Input: part model. Units: mm. Frame: model coordinates. A direction names the side the tool comes from. Coordinates: 2 decimals unless noted, no trailing zeros. Loops run counter-clockwise (first coordinate to the right, second up) from the corner with the lowest first, then second, coordinate; pieces in that order, holes last.
Autodesk Inventor part; units mm, degrees
ref_plane "YZ Plane" through (0, 0, 0) normal (1, 0, 0) x (0, 1, 0)
ref_plane "XZ Plane" through (0, 0, 0) normal (0, 1, 0) x (-1, 0, 0)
ref_plane "XY Plane" through (0, 0, 0) normal (0, 0, 1) x (1, 0, 0)
sketch "Sketch1" plane through (0, 0, 0) normal (0, 1, 0) x (-1, 0, 0)
  line L0 (0, 0) -> (14, 0)
  line L1 (14, 0) -> (14, -8.4)
  line L2 (14, -8.4) -> (0, -8.4)
  line L3 (0, -8.4) -> (0, 0)
  dimension "d0" = 8.4
  dimension "d1" = 14
extrude "Extrusion1" add sketch "Sketch1" along normal blind 2.5
sketch "Sketch2" plane through (0, 2.5, 0) normal (0, 1, 0) x (1, 0, 0)
  line L0 (-14, 2.85) -> (-5, 2.85)
  line L1 (-5, 5.55) -> (-14, 5.55)
  line L2 (-14, 5.55) -> (-14, 2.85)
  line L3 (-14, 8.4) -> (-14, 0)
  line L4 (-5, 2.85) -> (-5, 0)
  line L5 (-14, 0) -> (0, 0)
  line L6 (-5, 0) -> (0, 0)
  line L7 (0, 0) -> (0, 8.4)
  line L8 (0, 0) -> (0, 8.4)
  line L9 (-5, 5.55) -> (-5, 8.4)
  line L10 (0, 8.4) -> (-14, 8.4)
  point P0 (-14, 4.2)
  point P1 (-14, 4.2)
  point P2 (-5, 1.425)
  point P3 (-5, 6.975)
  dimension "d4" = 9
extrude "Extrusion2" add sketch "Sketch2" along normal blind 10 contours L2 L1 L9 L10 L7 L5 L4 L0
sketch "Sketch3" plane through (0, 0, 0) normal (0, -1, 0) x (1, 0, 0)
  line L0 (0, -29.6) -> (8, -29.6)
  line L1 (8, -29.6) -> (8, 21.2)
  line L2 (8, 21.2) -> (0, 21.2)
  line L3 (0, 21.2) -> (0, -29.6)
  line L4 (0, 0) -> (0, -8.4)
  point P0 (8, -4.2)
  point P1 (0, -4.2)
  point P2 (0, -4.2)
  dimension "d8" = 50.8
  dimension "d9" = 8
extrude "Extrusion3" add sketch "Sketch3" against normal up to surface (12.5 mm away)
sketch "Sketch4" plane through (0, 12.5, 0) normal (0, 1, 0) x (1, 0, 0)
  line L0 (16.1115, -33.9) -> (-34.6885, -33.9)
  line L1 (-34.6885, -33.9) -> (-34.6885, 42.3)
  line L2 (-34.6885, 42.3) -> (16.1115, 42.3)
  line L3 (16.1115, 42.3) -> (16.1115, -33.9)
  line L4 (8, 29.6) -> (8, -21.2)
  point P0 (0, 0)
  point P1 (16.1115, 4.2)
  point P2 (8, 4.2)
  dimension "d12" = 50.8
  dimension "d13" = 76.2
extrude "Extrusion4" add sketch "Sketch4" along normal blind 5
Item 1: Line query: L1, parallel to X at y = 10.5, z = 2.5; L2, parallel to Y at x = 13, z = 22; L3, parallel to X at y = 9.25, z = -7. Output: solid intervals per line, ascending.
Result:
L1: x = 0 to 8
L2: y = 12.5 to 17.5
L3: x = -5 to 8
Item 2: Section query B-B (y = 9.25). Output: boundary loops of the cut face in (x, z), then the cut area to 3 significant figures.
Result:
outline: (-14, -5.55) - (-5, -5.55) - (-5, -8.4) - (0, -8.4) - (0, -29.6) - (8, -29.6) - (8, 21.2) - (0, 21.2) - (0, 0) - (-5, 0) - (-5, -2.85) - (-14, -2.85) - close
area: 473 mm2
Item 3: Reachability of faces 1 (the face through (8, 6, -5)), 2 (the face through (-4, 5, -8.4)), 3 (the face through (4, 6, 21.2)), 4 (the face through (-4, 5, 0)) from +Z, -Z, +X, -X, +Y, -Y: full face, straight path, thin tool, end or side. Return the list, or none.
Result:
face 1: +Z, -Z, +X, -Y
face 2: -Z, -X, -Y
face 3: +Z, +X, -X, -Y
face 4: +Z, -X, -Y
Item 4: Section query C-C (z = -22). Output: boundary loops of the cut face in (x, y), then the cut area to 3 significant figures.
Result:
outline: (-34.69, 12.5) - (0, 12.5) - (0, 0) - (8, 0) - (8, 12.5) - (16.11, 12.5) - (16.11, 17.5) - (-34.69, 17.5) - close
area: 354 mm2
Item 5: Section query A-A (x = -1). Output: boundary loops of the cut face in (y, z), then the cut area to 3 significant figures.
Result:
outline: (0, -8.4) - (12.5, -8.4) - (12.5, -42.3) - (17.5, -42.3) - (17.5, 33.9) - (12.5, 33.9) - (12.5, 0) - (0, 0) - close
area: 486 mm2
Item 6: Section query D-D (x = -21). Output: boundary loops of the cut face in (y, z).
Result:
outline: (12.5, -42.3) - (17.5, -42.3) - (17.5, 33.9) - (12.5, 33.9) - close
Item 7: Contact query for flat-ended pins moving along their axis: P1, Ø5, axis at x = -5.5, z = -33.5, coming from the -Y side; P2, Ø9, axis at x = 2.5, y = 8.5, coming from the +Z side; P3, Ø10, axis at y = 4.5, z = 15.5, coming from the -X side; P4, Ø1, axis at x = 9.5, y = 5, coming from the -Z side. Output: stop coordinate, or through.
Result:
P1: stops at y = 12.5
P2: stops at z = 33.9
P3: stops at x = 0
P4: passes through
Item 8: Mould query, pull axis Y, two halves, no side actions, for faces 5 (the face through (2, 0, -4)), 6 (the face through (-14, 5, -4)), 7 (the face through (-9, 2.5, -7)), 8 (the face through (-10, 17.5, -5)). Classes: +Y half, -Y half, draft (parallel to the pull), parting line (faces both ways), or undercut.
Result:
face 5: -Y half
face 6: draft
face 7: undercut
face 8: +Y half
